Design review of the part shown in the three views and the two pictorial views. Dimensions are in mm from the part's minimum x, y and z. Round coordinates to 2 decimals unless told otherwise and drop trailing zeros. Loops run counter-clockwise (first coordinate to the right, second up) from the corner with the lowest first, then second, coordinate; pieces in that order, holes last.
1. To check wall thickness, follow line 1 along Z through (x, y) = (76.2, 4.75); line 2 along X through (y, z) = (3.5, 36.5); line 3 along X through (y, z) = (5.25, 110.5). State the ranges of each line that lie inside material, in increasing order.
2. Consider section D-D on x = 135. State the section outline as (y, z) points.
3. Consider section A-A on x = 76.2. State the section outline as (y, z) points.
4. Clearance check with flat-ended pins moving along their axes: pin 1 Ø5 at (y, z) = (3, 10.5) entering from +X; pin 2 Ø5 at (x, y) = (9, 4.5) entering from +Z; pin 3 Ø7 at (y, z) = (6.5, 141.5) entering from -X. State where each tip first meets the part, or that it passes through.
5. Consider section B-B on y = 10.75. State how many separate pieces and enclosed holes the cut face has, then the cut area to 3 significant figures.
6. Consider section C-C on z = 56.5. State the section outline as (x, y) points, then the cut area to 3 significant figures.
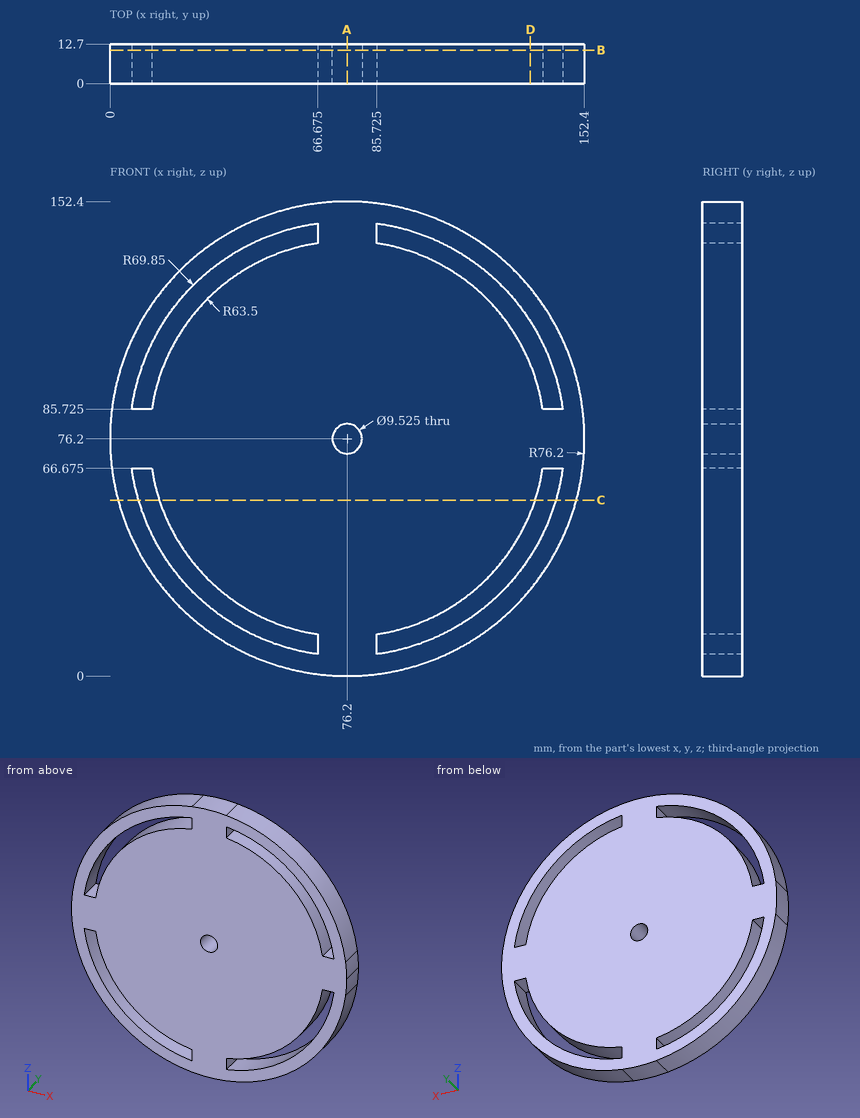
Resolved:
1. line 1: z = 0 to 71.44, 80.96 to 152.4
1. line 2: x = 11.16 to 18.73, 26.64 to 125.76, 133.67 to 141.24
1. line 3: x = 8.16 to 15.35, 22.76 to 129.64, 137.05 to 144.24
2. outline: (0, 27.73) - (12.7, 27.73) - (12.7, 38.5) - (0, 38.5) - close; (0, 52.22) - (12.7, 52.22) - (12.7, 100.18) - (0, 100.18) - close; (0, 113.9) - (12.7, 113.9) - (12.7, 124.67) - (0, 124.67) - close
3. outline: (0, 0) - (12.7, 0) - (12.7, 71.44) - (0, 71.44) - close; (0, 80.96) - (12.7, 80.96) - (12.7, 152.4) - (0, 152.4) - close
4. pin 1: stops at x = 118.77
4. pin 2: stops at z = 116.45
4. pin 3: stops at x = 31.62
5. separate pieces: 1
5. enclosed holes: 5
5. area: 16,000 mm2
6. outline: (2.59, 0) - (9.19, 0) - (9.19, 12.7) - (2.59, 12.7) - close; (15.83, 0) - (136.57, 0) - (136.57, 12.7) - (15.83, 12.7) - close; (143.21, 0) - (149.81, 0) - (149.81, 12.7) - (143.21, 12.7) - close
6. area: 1,700 mm2
